The listing builds one solid part. Answer for the finished solid, in the listing's coordinates (mm). A direction names the side the tool comes from. Give positions to 0.01 mm unless a question says otherwise; leave off trailing zeros. Write each loop counter-clockwise with the first axis right and the second up, starting at its lowest first coordinate (ties: lowest second). Pieces come first, ordered by that corner, then holes. Notation, with made-up numbers: M -9.75,-32.75 L 44.25,-32.75 A34 ccw 44.25,5.25 Z; hole C 15,30.5 d6. An arc over 180 degrees is marked long. Answer as a JSON object with one key per item and string values.
Autodesk Inventor part; units mm, degrees
ref_plane "YZ Plane" through (0, 0, 0) normal (1, 0, 0) x (0, 1, 0)
ref_plane "XZ Plane" through (0, 0, 0) normal (0, 1, 0) x (-1, 0, 0)
ref_plane "XY Plane" through (0, 0, 0) normal (0, 0, 1) x (1, 0, 0)
sketch "Szkic1" plane through (0, 0, 0) normal (0, 0, 1) x (1, 0, 0)
  line L0 (0, 0) -> (-10, 0)
  line L1 (-10, 0) -> (-10, 32.68)
  line L2 (-10, 32.68) -> (0, 32.68)
  line L3 (0, 32.68) -> (0, 0)
  arc A0 (0, 32.68) -> (-10, 32.68) centre (-5, 32.68) ccw
  circle A1 centre (-5, 32.68) radius 3
  dimension "d2" = 10
  dimension "d3" = 32.68
  dimension "d4" = 6
extrude "Wyciągnięcie proste1" add sketch "Szkic1" against normal blind 10 contours L0 L1 L2 A1 L3 | L2 A1 A0
sketch "Szkic2" plane through (-10, 0, 0) normal (-1, 0, 0) x (0, 0, 1)
  line L0 (-10, 29.68) -> (0, 29.68)
  line L1 (-13.2063, 25.68) -> (3.6302, 25.68)
  line L2 (0, 32.68) -> (-10, 32.68)
  line L3 (-5, 32.68) -> (-5, 38.3797)
  line L4 (-7, 25.68) -> (-3, 25.68)
  line L5 (-3, 25.68) -> (-3, 38.3797)
  line L6 (-3, 38.3797) -> (-7, 38.3797)
  line L7 (-7, 38.3797) -> (-7, 25.68)
  point P0 (0, 0)
  dimension "d7" = 7
  dimension "d8" = 4
extrude "Wyciągnięcie proste2" cut sketch "Szkic2" against normal blind 10
sketch "Szkic3" plane through (-10, 0, 0) normal (0, -1, 0) x (1, 0, 0)
  line L0 (0, -10) -> (10, -10)
  line L1 (5, -10) -> (5, 0)
  line L2 (0, 0) -> (10, 0)
  line L3 (10, 0) -> (10, -10)
  line L4 (10, -5) -> (0, -5)
  line L5 (0, 0) -> (0, -10)
  point P0 (5, -5)
hole "Otwór1" at (-5, 0, -5) direction (0, 1, 0) diameter 2.459 depth 8.8 tip angle 118
sketch "Szkic4" plane through (-10, 0, 0) normal (0, -1, 0) x (1, 0, 0)
  line L0 (10, 0) -> (10, -10)
  line L1 (0, 0) -> (0, -10)
  line L2 (10, -10) -> (0, -10)
  line L3 (0, -10) -> (0, 0)
  line L4 (0, 0) -> (10, 0)
  line L5 (10, 0) -> (10, -10)
  circle A0 centre (5, -5) radius 1.2295
  circle A1 centre (5, -5) radius 5
  point P0 (0, -5)
  point P1 (5, 0)
  point P2 (10, -5)
  point P3 (5, -10)
extrude "Wyciągnięcie proste3" cut sketch "Szkic4" against normal blind 22.68 contours L0 A1 L4 | L0 L2 A1 | A1 L1 L4 | L2 L1 A1
properties part number "Część L5" material "Stal nierdzewna 440C"
1. The mould has two halves that part along Z. Classify faces 4 (the flat face through (-5, 29, 0)), 5 (the conical face through (-4.82, 9.41, -5.11)), 6 (the flat face through (-9, 22.68, -9)): released by +Z, released by -Z, zero draft, split by the parting line, or undercut.
Verdict:
{"face 4": "released by +Z", "face 5": "undercut", "face 6": "zero draft"}
2. A cutting plane is placed at C-C, the plane x = -9. Give the vertices of the cut face in (y, z).
Verdict:
{"outline": "M 0,-8 L 22.68,-8 L 22.68,-10 L 35.68,-10 L 35.68,-7 L 25.68,-7 L 25.68,-3 L 35.68,-3 L 35.68,0 L 22.68,0 L 22.68,-2 L 0,-2 Z"}
3. For faces 1 (the cylindrical face through (-4.252, 4.462, -4.024)), 2 (the flat face through (-1, 22.68, -1)), 3 (the flat face through (-5, 29, -3)), determine the directions among +Z, -Z, +X, -X, +Y, -Y from which every point of the face is accessible in a straight line to the end or side of a thin tool.
Verdict:
{"face 1": "-Y", "face 2": "+Z, +X, -Y", "face 3": "+X, -X, +Y"}
4. A cutting plane is placed at B-B, the plane y = 34.5. Give the vertices of the cut face in (x, z), plus the area to 3 significant figures.
Verdict:
{"outline": "M -9.66,-10 L -7.38,-10 L -7.38,-7 L -9.66,-7 Z; M -9.66,-3 L -7.38,-3 L -7.38,0 L -9.66,0 Z; M -2.62,-10 L -0.34,-10 L -0.34,-7 L -2.62,-7 Z; M -2.62,-3 L -0.34,-3 L -0.34,0 L -2.62,0 Z", "area": "27.3 mm2"}
5. Flat-ended cylindrical pins translate along their axes: pin 1 (5 mm diameter, centred on x = -5, y = 32.68, fed in from -Z); pin 2 (2 mm diameter, centred on y = 9, z = -2.5, fed in from -X); pin 3 (1.2 mm diameter, centred on x = -6.5, z = -4, fed in from +Y). Find the tip coordinate at first contact, or state that the pin passes through.
Verdict:
{"pin 1": "passes through", "pin 2": "stops at x = -9.77", "pin 3": "stops at y = 25.68"}
6. A cutting plane is placed at D-D, the plane z = -7.5. Give the vertices of the cut face in (x, y), plus the area to 3 significant figures.
Verdict:
{"outline": "M -10,22.68 L -9.33,22.68 L -9.33,0 L -0.67,0 L -0.67,22.68 L 0,22.68 L 0,32.68 A5 ccw -10,32.68 Z; hole C -5,32.68 d6", "area": "307 mm2"}
7. Consider line 1 along Z through (x, y) = (-5, 7); line 2 along Z through (x, y) = (-1.75, 35). Determine where each line is inside the solid, lowest interval first.
Verdict:
{"line 1": "z = -10 to -6.23, -3.77 to 0", "line 2": "z = -10 to -7, -3 to 0"}
8. A cutting plane is placed at A-A, the plane y = 26.5. Give the vertices of the cut face in (x, z).
Verdict:
{"outline": "M -10,-10 L 0,-10 L 0,-7 L -10,-7 Z; M -10,-3 L 0,-3 L 0,0 L -10,0 Z"}
